from build123d import *

# Parameters (mm, degrees)
F0_W     = 215.9
F0_H     = 25.4
F1_DEPTH = 25.4
F2_DEPTH = 12.7
F3_SIZE2 = 25.39999
F3_SIZE  = 25.39999


# Not quite as in the source:
# - a fillet or chamfer is up to 0.001 mm smaller than in the source, because OpenCascade refuses the exact size


with BuildPart() as f1:
    # F0 (on Front) → F1 (new body)
    with BuildSketch(Plane.XZ):
        with Locations((-71.4832603614, 24.0690046921)):
            Rectangle(F0_W, F0_H)
    extrude(amount=-F1_DEPTH)

    # F2 (add): a face of the model
    f2_faces = [f1.faces().sort_by_distance(p)[0] for p in [
        (36.4667396386, 12.7, 24.0690046921),
    ]]
    extrude(f2_faces, amount=F2_DEPTH)

    # F3 (size 25.4 and 25.4 in the source; OpenCascade refuses exactly that, so slightly less here)
    f3_edges = [f1.edges().sort_by_distance(p)[0] for p in [
        (-179.43326, 12.7, 11.369005),
    ]]
    chamfer(f3_edges, length=F3_SIZE, length2=F3_SIZE2)


solid = f1.part
Geometry check sheet. Reference: the model listing, model coordinates, mm. Give positions to 0.01 mm unless a question says otherwise; leave off trailing zeros. Order: outer loops, then holes, each group sorted by start corner. A loop starts at its lowest first (then second) coordinate and runs counter-clockwise, first axis right, second up. Notation, with made-up numbers: (51, -7.5) - (86, -7.5) arc R27 cw to (86, 31.5) - close; hole circle Ø8 at (60, 55.5). An arc over 180 degrees is marked (long way). Answer as a JSON object with one key per item and string values.
(1) Depth check by flat-ended pin: pin 1 Ø3 at (y, z) = (19, 30.5) entering from -X. Enter the tip coordinate at first touch or a pass-through.
Report:
{"pin 1": "x = -174.66"}
(2) Cross-section at C-C (z = 28.75). Record the cut outline in (x, y).
Report:
{"outline": "(-171.41, 0) - (49.17, 0) - (49.17, 25.4) - (-171.41, 25.4) - close"}
(3) Cross-section at B-B (x = -162). Record the cut outline in (y, z), then the cut area to 3 significant figures.
Report:
{"outline": "(0, 19.34) - (25.4, 19.34) - (25.4, 36.77) - (0, 36.77) - close", "area": "443 mm^2"}
(4) Material ranges on line 1 (X direction, y = 21, z = 25.5); line 2 (X direction, y = 6, z = 16), recorded low to high.
Report:
{"line 1": "-168.16 to 49.17", "line 2": "-158.66 to 49.17"}
